Answer from the drawing. Dimensions are ordinates in mm from the lowest x, y and z of the part. A direction names the side the tool comes from. Coordinates: 2 decimals unless noted, no trailing zeros. Order: outer loops, then holes, each group sorted by start corner. A loop starts at its lowest first (then second) coordinate and runs counter-clockwise, first axis right, second up.
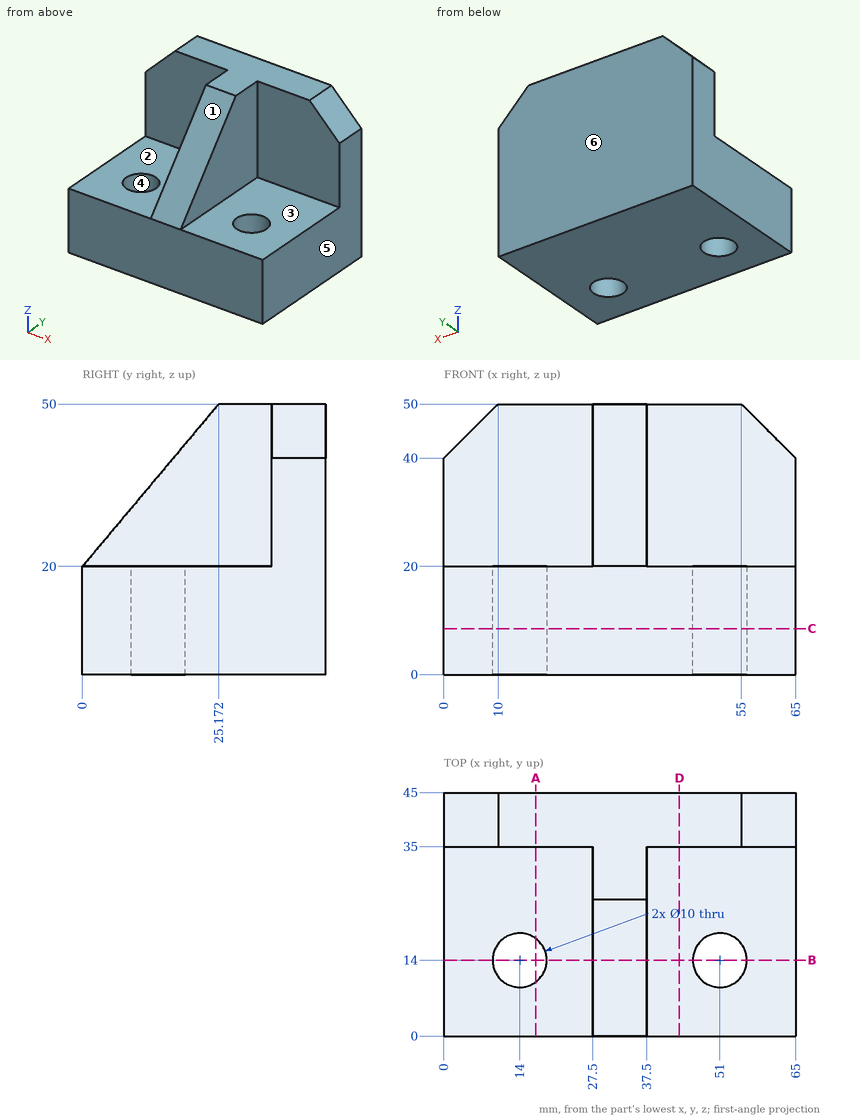
1. The part is cut by section A-A (x = 17). Determine the outline of the cut face in (y, z).
2. Consider probe 1 along Y at (x, z) = (14, 11.5); probe 2 along Z at (x, y) = (20.5, 25); probe 3 along X at (y, z) = (34.5, 38). Determine where each line is inside the solid, lowest interval first.
3. The part is cut by section B-B (y = 14). Determine the outline of the cut face in (x, z) (1 decimal).
4. The mould has two halves that part along Y. Classify the marked faces 4, 5 and 6: released by +Y, released by -Y, zero draft, split by the parting line, or undercut.
5. Flat-ended cylindrical pins translate along their axes: pin 1 (10 mm diameter, centred on x = 50.5, z = 27, fed in from -Y); pin 2 (1 mm diameter, centred on x = 32.5, z = 34, fed in from -Y); pin 3 (15 mm diameter, centred on y = 19, z = 36, fed in from +X); pin 4 (8 mm diameter, centred on x = 9, y = 15.5, fed in from -Z). Find the tip coordinate at first contact, or state that the pin passes through.
6. The part is cut by section D-D (x = 43.5). Determine the outline of the cut face in (y, z), plus the area to 3 significant figures.
7. For the marked faces 1, 2 and 3, determine the directions among +Z, -Z, +X, -X, +Y, -Y from which every point of the face is accessible in a straight line to the end or side of a thin tool.
8. The part is cut by section C-C (z = 8.5). Determine the outline of the cut face in (x, y).
Worked out:
1. outline: (0, 0) - (10, 0) - (10, 20) - (0, 20) - close; (18, 0) - (45, 0) - (45, 50) - (35, 50) - (35, 20) - (18, 20) - close
2. probe 1: y = 0 to 9, 19 to 45
2. probe 2: z = 0 to 20
2. probe 3: x = 27.5 to 37.5
3. outline: (0, 0) - (9, 0) - (9, 20) - (0, 20) - close; (19, 0) - (46, 0) - (46, 20) - (37.5, 20) - (37.5, 36.7) - (27.5, 36.7) - (27.5, 20) - (19, 20) - close; (56, 0) - (65, 0) - (65, 20) - (56, 20) - close
4. face 4: undercut
4. face 5: zero draft
4. face 6: released by +Y
5. pin 1: stops at y = 35
5. pin 2: stops at y = 11.33
5. pin 3: stops at x = 37.5
5. pin 4: stops at z = 0
6. outline: (0, 0) - (45, 0) - (45, 50) - (35, 50) - (35, 20) - (0, 20) - close
6. area: 1,200 mm2
7. face 1: +Z, +X, -X, -Y
7. face 2: +Z, -X, -Y
7. face 3: +Z, +X, -Y
8. outline: (0, 0) - (65, 0) - (65, 45) - (0, 45) - close; hole circle Ø10 at (14, 14); hole circle Ø10 at (51, 14)
